The model under review builds one solid part; all positions refer to its coordinate system, in mm. Round coordinates to 2 decimals unless told otherwise and drop trailing zeros. Order: outer loops, then holes, each group sorted by start corner. A loop starts at its lowest first (then second) coordinate and runs counter-clockwise, first axis right, second up. Notation, with made-up numbers: M 20,13 L 56,13 A8 cw 56,20 Z; hole C -7.75,45.25 d2. An arc over 180 degrees is marked long. Answer as a JSON object with one key per item and string values. Group by question number.
1. To check wall thickness, follow probe 1 along X at (y, z) = (-29, 1.1); probe 2 along Y at (x, z) = (-50.5, 0.35); probe 3 along Y at (x, z) = (-11, 2.85). State the ranges of each line that lie inside material, in increasing order. Write a range as [from, to].
2. Add section A-A on x = -32. State the section outline as (y, z) points.
3. Add section C-C on z = 1.85. State the section outline as (x, y) points.
4. Add section B-B on x = -53.5. State the section outline as (y, z) points.
5. Clearance check with a flat-ended pin moving along its axis: P1, Ø6, axis at x = -13.23, y = 11.16, coming from the +Z side. State where the tip first meets the part, or that it passes through.
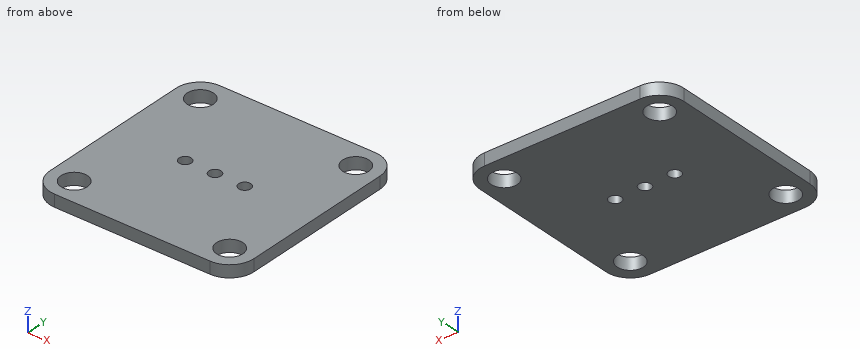
```python
from build123d import *

# Parameters (mm, degrees)
F0_R     = 3.25
F0_R_2   = 1.5
F1_DEPTH = 3


with BuildPart() as f1:
    # F0 (on Top) → F1 (new body)
    with BuildSketch(Plane.XY):
        with BuildLine():
            Line((-13.232693, 17.157822), (-51.732693, 17.157822))
            ThreePointArc((-51.732693, 17.157822), (-55.975334, 15.400463), (-57.732693, 11.157822))
            Line((-57.732693, 11.157822), (-57.732693, -27.342178))
            ThreePointArc((-57.732693, -27.342178), (-55.975334, -31.584819), (-51.732693, -33.342178))
            Line((-51.732693, -33.342178), (-13.232693, -33.342178))
            ThreePointArc((-13.232693, -33.342178), (-8.990052, -31.584819), (-7.232693, -27.342178))
            Line((-7.232693, -27.342178), (-7.232693, 11.157822))
            ThreePointArc((-7.232693, 11.157822), (-8.990052, 15.400463), (-13.232693, 17.157822))
        make_face()
        with Locations((-51.732693, -27.342178)):
            Circle(F0_R, mode=Mode.SUBTRACT)
        with Locations((-39.862693, -8.092178)):
            Circle(F0_R_2, mode=Mode.SUBTRACT)
        with Locations((-32.482693, -8.092178)):
            Circle(F0_R_2, mode=Mode.SUBTRACT)
        with Locations((-13.232693, -27.342178)):
            Circle(F0_R, mode=Mode.SUBTRACT)
        with Locations((-25.102693, -8.092178)):
            Circle(F0_R_2, mode=Mode.SUBTRACT)
        with Locations((-51.732693, 11.157822)):
            Circle(F0_R, mode=Mode.SUBTRACT)
        with Locations((-13.232693, 11.157822)):
            Circle(F0_R, mode=Mode.SUBTRACT)
    extrude(amount=F1_DEPTH)


solid = f1.part
```
Recorded:
{
 "1": {"probe 1": "x = [-57.5, -54.53], [-48.94, -16.03], [-10.44, -7.47]", "probe 2": "y = [-33.34, -30.35], [-24.34, 8.15], [14.16, 17.16]", "probe 3": "y = [-32.91, -29.7], [-24.98, 8.8], [13.52, 16.73]"},
 "2": {"outline": "M -33.34,0 L -9.51,0 L -9.51,3 L -33.34,3 Z; M -6.67,0 L 17.16,0 L 17.16,3 L -6.67,3 Z"},
 "3": {"outline": "M -57.73,-27.34 A6 ccw -51.73,-33.34 L -13.23,-33.34 A6 ccw -7.23,-27.34 L -7.23,11.16 A6 ccw -13.23,17.16 L -51.73,17.16 A6 ccw -57.73,11.16 Z; hole C -51.73,-27.34 d6.5; hole C -51.73,11.16 d6.5; hole C -39.86,-8.09 d3; hole C -32.48,-8.09 d3; hole C -25.1,-8.09 d3; hole C -13.23,-27.34 d6.5; hole C -13.23,11.16 d6.5"},
 "4": {"outline": "M -33.08,0 L -30.07,0 L -30.07,3 L -33.08,3 Z; M -24.61,0 L 8.43,0 L 8.43,3 L -24.61,3 Z; M 13.89,0 L 16.89,0 L 16.89,3 L 13.89,3 Z"},
 "5": {"P1": "passes through"}
}
